from build123d import *

# Parameters (mm, degrees)
SKETCH1_W            = 101.6
SKETCH1_H            = 37
BASE_SHAPE_DEPTH     = 2.4638
SKETCH2_R            = 6
SKETCH2_R_2          = 1.75
MOTOR_HOLES_DEPTH    = 55.11986983
SKETCH4_W            = 19.05
SKETCH4_H            = 2.4638
BOTTOM_TEETH_DEPTH   = 5.334
SKETCH5_W            = 5.334
SKETCH5_H            = 12.7
SIDE_SLOTS_DEPTH     = 57.167338075
SKETCH7_W            = 15.24
SKETCH7_H            = 12.7
ENCODER_CUTOUT_DEPTH = 72.809068434
SKETCH8_R            = 1.5
ENCODER_MOUNTS_DEPTH = 57.167338075


with BuildPart() as part:
    # Sketch1 → Base Shape (new body)
    with BuildSketch(Plane.XY):
        Rectangle(SKETCH1_W, SKETCH1_H)
    extrude(amount=-BASE_SHAPE_DEPTH)

    # Sketch2 → Motor Holes (cut, through all)
    with BuildSketch(Plane.XY):
        with Locations((0, -8.73)):
            Circle(SKETCH2_R)
        with Locations((-10.25, -8.73)):
            Circle(SKETCH2_R_2)
        with Locations((10.25, -8.73)):
            Circle(SKETCH2_R_2)
        with Locations((0, 13.369999996)):
            Circle(SKETCH2_R_2)
    extrude(amount=-MOTOR_HOLES_DEPTH, mode=Mode.SUBTRACT)

    # Sketch4 → Bottom teeth (add)
    with BuildSketch(Plane.XZ.offset(18.5)):
        with Locations((-41.275, -1.2319)):
            Rectangle(SKETCH4_W, SKETCH4_H)
        with Locations((0, -1.2319)):
            Rectangle(SKETCH4_W, SKETCH4_H)
        with Locations((41.275, -1.2319)):
            Rectangle(SKETCH4_W, SKETCH4_H)
    extrude(amount=BOTTOM_TEETH_DEPTH)

    # Sketch5 → Side Slots (cut, through all)
    with BuildSketch(Plane.XY):
        with Locations((48.133, 0)):
            Rectangle(SKETCH5_W, SKETCH5_H)
        with Locations((-48.133, 0)):
            Rectangle(SKETCH5_W, SKETCH5_H)
    extrude(amount=-SIDE_SLOTS_DEPTH, mode=Mode.SUBTRACT)

    # Sketch7 → Encoder Cutout (cut, through all)
    with BuildSketch(Plane(origin=(16.243120564, -7.106483242, 0), x_dir=(1, 0, 0), z_dir=(0, 0, 1))):
        with Locations((15.252879436, 0.290483242)):
            Rectangle(SKETCH7_W, SKETCH7_H)
    extrude(amount=-ENCODER_CUTOUT_DEPTH, mode=Mode.SUBTRACT)

    # Sketch8 → Encoder Mounts (cut, through all)
    with BuildSketch(Plane.XY):
        with Locations((31.496, 2.074)):
            Circle(SKETCH8_R)
        with Locations((31.496, -15.706)):
            Circle(SKETCH8_R)
    extrude(amount=-ENCODER_MOUNTS_DEPTH, mode=Mode.SUBTRACT)


solid = part.part
Input: part model. Units: mm. Frame: model coordinates. A direction names the side the tool comes from. Give positions to 0.01 mm unless a question says otherwise; leave off trailing zeros. Write each loop counter-clockwise with the first axis right and the second up, starting at its lowest first coordinate (ties: lowest second). Pieces come first, ordered by that corner, then holes.
Q1. Material intervals for probe 1 along X at (y, z) = (-9, -2); probe 2 along Y at (x, z) = (0, -0.9); probe 3 along Y at (x, z) = (-10.25, -1.55), sorted ascending.
Q2. Section C-C, the plane x = 38. Output: boundary loops of the cut face in (y, z), plus the area to 3 significant figures.
Q3. Section B-B, the plane x = 0. Output: boundary loops of the cut face in (y, z), plus the area to 3 significant figures.
Q4. First-contact query: P1, Ø4, axis at x = 10.25, y = -8.73, coming from the -Z side; P2, Ø7, axis at x = 0, y = -8.73, coming from the +Z side; P3, Ø1.2, axis at y = 0.5, z = -1, coming from the +X side. Flat tips, straight axial feed; report the tip coordinate or a pass-through.
Q5. Section A-A, the plane y = -20. Output: boundary loops of the cut face in (x, z) (3 decimals), plus the area to 3 significant figures.
Q6. Set-up query: faces 1 (the face through (-1, 18.5, -1)), 2 (the face through (-48, 6.35, -1)), 3 (the face through (48, 6.35, -1)), 4 (the face through (-31.75, -21, -1)), 5 (the face through (39.116, -7, -1)). Return all of +Z, -Z, +X, -X, +Y, -Y with unobstructed straight access to the full face (end or side cutting, diameter ignored); none if empty.
Q7. Section D-D, the plane y = 13.37. Output: boundary loops of the cut face in (x, z), plus the area to 3 significant figures.
Q8. Pull-direction query (Y, two-part tool) for faces 6 (the face through (-50.8, -15, -1)), 7 (the face through (-21, -18.5, -1)), 8 (the face through (-48, -6.35, -1)); classes: pulls with the +Y half, pulls with the -Y half, needs draft (parallel to the pull), parting line crosses it, or undercut.
Filled in:
1. probe 1: x = -50.8 to -11.98, -8.52 to -5.99, 5.99 to 8.52, 11.98 to 23.88, 39.12 to 50.8
1. probe 2: y = -23.83 to -14.73, -2.73 to 11.62, 15.12 to 18.5
1. probe 3: y = -18.5 to -10.48, -6.98 to 18.5
2. outline: (-23.83, -2.46) - (-13.17, -2.46) - (-13.17, 0) - (-23.83, 0) - close; (-0.47, -2.46) - (18.5, -2.46) - (18.5, 0) - (-0.47, 0) - close
2. area: 73.0 mm2
3. outline: (-23.83, -2.46) - (-14.73, -2.46) - (-14.73, 0) - (-23.83, 0) - close; (-2.73, -2.46) - (11.62, -2.46) - (11.62, 0) - (-2.73, 0) - close; (15.12, -2.46) - (18.5, -2.46) - (18.5, 0) - (15.12, 0) - close
3. area: 66.1 mm2
4. P1: stops at z = -2.46
4. P2: passes through
4. P3: stops at x = 45.47
5. outline: (-50.8, -2.464) - (-31.75, -2.464) - (-31.75, 0) - (-50.8, 0) - close; (-9.525, -2.464) - (9.525, -2.464) - (9.525, 0) - (-9.525, 0) - close; (31.75, -2.464) - (50.8, -2.464) - (50.8, 0) - (31.75, 0) - close
5. area: 141 mm2
6. face 1: +Z, -Z, +X, -X, +Y
6. face 2: +Z, -Z, -X
6. face 3: +Z, -Z, +X
6. face 4: +Z, -Z, -Y
6. face 5: +Z, -Z
7. outline: (-50.8, -2.46) - (-1.75, -2.46) - (-1.75, 0) - (-50.8, 0) - close; (1.75, -2.46) - (50.8, -2.46) - (50.8, 0) - (1.75, 0) - close
7. area: 242 mm2
8. face 6: needs draft
8. face 7: pulls with the -Y half
8. face 8: undercut
